```python
from build123d import *

# Parameters (mm, degrees)
F0_R     = 11
F1_DEPTH = 3


with BuildPart() as f1:
    # F0 (on Top) → F1 (new body, symmetric)
    with BuildSketch(Plane.XY):
        with BuildLine():
            ThreePointArc((-2, 14.671401), (-2.560407, 12.925438), (-4.032258, 11.831775))
            ThreePointArc((-4.032258, 11.831775), (-10.411858, 6.916879), (-12.469754, -0.869041))
            ThreePointArc((-12.469754, -0.869041), (-12.787701, -2.097561), (-13.780875, -2.887473))
            Line((-13.780875, -2.887473), (-14.905284, -3.296724))
            ThreePointArc((-14.905284, -3.296724), (-42.286168, -15.390906), (-13.537203, -7.055495))
            Line((-13.537203, -7.055495), (-12.412794, -6.646243))
            ThreePointArc((-12.412794, -6.646243), (-11.144234, -6.61295), (-10.110995, -7.34968))
            ThreePointArc((-10.110995, -7.34968), (-0.850808, -12.471011), (9.019124, -8.654791))
            ThreePointArc((9.019124, -8.654791), (10.63235, -7.783043), (12.451568, -8.013017))
            Line((12.451568, -8.013017), (15.598444, -9.48043))
            ThreePointArc((15.598444, -9.48043), (41.690158, -19.44044), (17.288917, -5.855198))
            Line((17.288917, -5.855198), (14.142041, -4.387786))
            ThreePointArc((14.142041, -4.387786), (12.7965, -3.142009), (12.427336, -1.345857))
            ThreePointArc((12.427336, -1.345857), (10.542393, 6.716245), (4.032258, 11.831775))
            ThreePointArc((4.032258, 11.831775), (2.560407, 12.925438), (2, 14.671401))
            Line((2, 14.671401), (2, 29.661037))
            ThreePointArc((2, 29.661037), (0, 54.5), (-2, 29.661037))
            Line((-2, 29.661037), (-2, 14.671401))
        make_face()
        with Locations((-28.190779, -10.260604)):
            Circle(F0_R, mode=Mode.SUBTRACT)
        with Locations((29.001849, -13.523784)):
            Circle(F0_R, mode=Mode.SUBTRACT)
        Circle(F0_R, mode=Mode.SUBTRACT)
        with Locations((0, 42)):
            Circle(F0_R, mode=Mode.SUBTRACT)
    extrude(amount=F1_DEPTH, both=True)


solid = f1.part
```
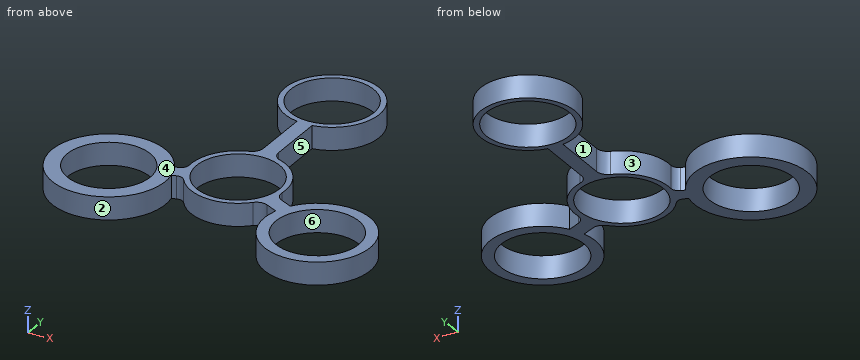
The model under review builds one solid part; all positions refer to its coordinate system, in mm. Face numbers are marked on the shaded views. A direction names the side the tool comes from. Round coordinates to 2 decimals unless told otherwise and drop trailing zeros. Write each loop counter-clockwise with the first axis right and the second up, starting at its lowest first coordinate (ties: lowest second). Pieces come first, ordered by that corner, then holes. Notation, with made-up numbers: (84.25, -1.75) - (105.25, -1.75) arc R30 cw to (105.25, 36.25) - close; hole circle Ø4 at (85, 81). An arc over 180 degrees is marked (long way). Use one line per item in the form item = value.
Q1. Consider section A-A (x = 0). State the section outline as (y, z) points.
Answer key:
outline = (-12.5, -3) - (-11, -3) - (-11, 3) - (-12.5, 3) - close; (11, -3) - (31, -3) - (31, 3) - (11, 3) - close; (53, -3) - (54.5, -3) - (54.5, 3) - (53, 3) - close
Q2. Consider section C-C (x = 25). State the section outline as (y, z) points.
Answer key:
outline = (-26.94, -3) - (-23.77, -3) - (-23.77, 3) - (-26.94, 3) - close; (-3.28, -3) - (-0.11, -3) - (-0.11, 3) - (-3.28, 3) - close
Q3. Draft analysis for pull direction X (two halves, no side actions). For the marked faces 3, 4, 5 and 6, state which applies: +X half, -X half, draft (parallel to the pull), parting line (faces both ways), or undercut.
Answer key:
face_3 = undercut
face_4 = draft
face_5 = +X half
face_6 = undercut
Q4. Consider section D-D (z = 2). State the section outline as (x, y) points, and give its area (3 significant figures).
Answer key:
outline = (-14.91, -3.3) arc R15 ccw (long way) to (-13.54, -7.06) - (-12.41, -6.65) arc R2 cw to (-10.11, -7.35) arc R12.5 ccw to (9.02, -8.65) arc R3 cw to (12.45, -8.01) - (15.6, -9.48) arc R14 ccw (long way) to (17.29, -5.86) - (14.14, -4.39) arc R3 cw to (12.43, -1.35) arc R12.5 ccw to (4.03, 11.83) arc R3 cw to (2, 14.67) - (2, 29.66) arc R12.5 ccw (long way) to (-2, 29.66) - (-2, 14.67) arc R3 cw to (-4.03, 11.83) arc R12.5 ccw to (-12.47, -0.87) arc R2 cw to (-13.78, -2.89) - close; hole circle Ø22 at (-28.19, -10.26); hole circle Ø22 at (0, 0); hole circle Ø22 at (0, 42); hole circle Ø22 at (29, -13.52)
area = 890 mm2
Q5. Tool access review of the marked faces 1 and 2: name each direction out of +Z, -Z, +X, -X, +Y, -Y from which nothing blocks a thin tool from reaching the whole face with its end or side.
Answer key:
face_1 = +Z, -Z, -X
face_2 = +Z, -Z
Q6. For line 1 (Y direction, x = 0, z = 0.7); line 2 (X direction, y = -2, z = 0.8); line 3 (Y direction, x = -8, z = 2.4), list the stretches that pass through material, from the lowest coordinate up. Write a range as [from, to].
Answer key:
line_1 = [-12.5, -11], [11, 31], [53, 54.5]
line_2 = [-40.71, -35.45], [-20.93, -15.67], [-12.73, -10.82], [10.82, 12.43], [21.05, 36.95]
line_3 = [-9.6, -7.55], [7.55, 9.6], [32.4, 34.45], [49.55, 51.6]
Q7. Insertion check: pin 1 Ø3 at (x, z) = (5.5, 0.5) entering from +Y; pin 2 Ø1 at (y, z) = (14, -1) entering from +X; pin 3 Ø2 at (y, z) = (4, 0.5) entering from -X. Each pin has a flat end and moves straight along its axis. Give the tip position at first contact, or say it passes through.
Answer key:
pin_1 = 53.84
pin_2 = 2.24
pin_3 = -35.2
Q8. Consider section B-B (y = 42). State the section outline as (x, z) points, and give its area (3 significant figures).
Answer key:
outline = (-12.5, -3) - (-11, -3) - (-11, 3) - (-12.5, 3) - close; (11, -3) - (12.5, -3) - (12.5, 3) - (11, 3) - close
area = 18.0 mm2
